The figure shows three views and two pictorial views of one solid part (mm, origin at its lowest corner). Answer the questions. A direction names the side the tool comes from. Round coordinates to 2 decimals unless told otherwise and drop trailing zeros. Write each loop counter-clockwise with the first axis right and the second up, starting at its lowest first coordinate (ties: lowest second). Pieces come first, ordered by that corner, then holes. Notation, with made-up numbers: (-2, -20) -> (14, -20) arc R27 cw to (14, 7) -> close; hole circle Ø2 at (60.25, -34.5). An arc over 180 degrees is marked (long way). One line per item, written item: value.
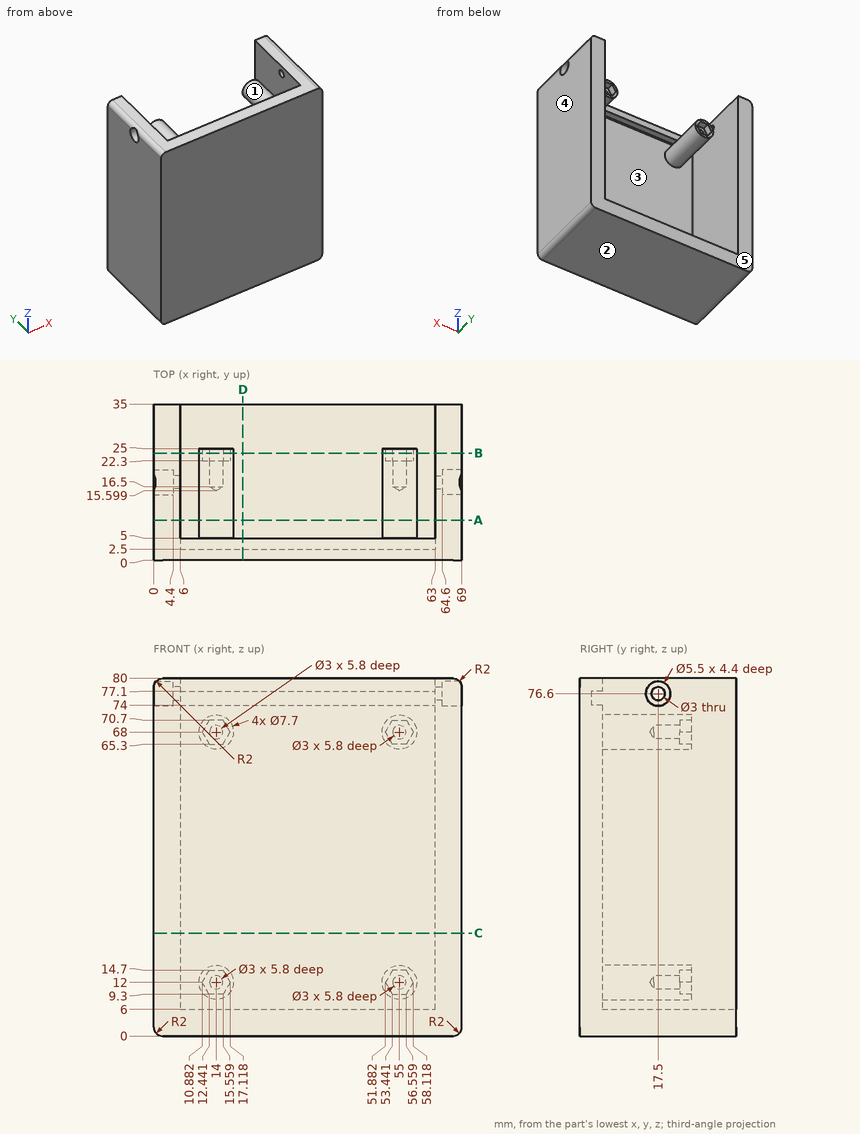
(1) Flat-ended cylindrical pins translate along their axes: pin 1 Ø5 at (y, z) = (17.5, 76.6) entering from -X; pin 2 Ø1.3 at (x, y) = (14.5, 23.5) entering from +Z; pin 3 Ø2.5 at (x, z) = (56.5, 66.5) entering from +Y. Find the tip coordinate at first contact, or state that the pin passes through.
Reported:
pin 1: stops at x = 4.4
pin 2: stops at z = 71.85
pin 3: stops at y = 25
(2) For a pull along X with two mould halves and no side action, classify the marked faces 3, 4 and 5 as pulls with the +X half, pulls with the -X half, needs draft (parallel to the pull), parting line crosses it, or undercut.
Reported:
face 3: undercut
face 4: pulls with the +X half
face 5: needs draft
(3) Find section B-B on y = 24. Give the number of separate pieces and of enclosed holes in the cut face, plus the area to 3 significant figures.
Reported:
separate pieces: 5
enclosed holes: 4
area: 1,380 mm2
(4) A tool of negligible diameter and unlimited length cuts with its end or side. For the marked faces 1 and 2, from which of +Z, -Z, +X, -X, +Y, -Y can it reach the whole face along a straight path? Write none if from no direction.
Reported:
face 1: +Y
face 2: -Z, +X, -X, +Y, -Y
(5) Find section A-A on y = 9. Give the vertices of the cut face in (x, z).
Reported:
outline: (0, 2) arc R2 ccw to (2, 0) -> (67, 0) arc R2 ccw to (69, 2) -> (69, 78) arc R2 ccw to (67, 80) -> (63, 80) -> (63, 6) -> (6, 6) -> (6, 80) -> (2, 80) arc R2 ccw to (0, 78) -> close; circle Ø7.7 at (14, 12); circle Ø7.7 at (14, 68); circle Ø7.7 at (55, 12); circle Ø7.7 at (55, 68)
(6) Find section C-C on z = 23. Give the vertices of the cut face in (x, y), plus the area to 3 significant figures.
Reported:
outline: (0, 0) -> (69, 0) -> (69, 35) -> (63, 35) -> (63, 5) -> (6, 5) -> (6, 35) -> (0, 35) -> close
area: 705 mm2
(7) Find section D-D on x = 20. Give the vertices of the cut face in (y, z), plus the area to 3 significant figures.
Reported:
outline: (0, 0) -> (35, 0) -> (35, 6) -> (5, 6) -> (5, 74) -> (2.5, 74) -> (2.5, 77.1) -> (5, 77.1) -> (5, 80) -> (0, 80) -> close
area: 572 mm2
(8) Consider probe 1 along X at (y, z) = (19.75, 68); probe 2 along X at (y, z) = (14, 50.5); probe 3 along Y at (x, z) = (1.85, 76.6). Determine where each line is inside the solid, lowest interval first.
Reported:
probe 1: x = 0 to 6, 10.15 to 12.5, 15.5 to 17.85, 51.15 to 53.5, 56.5 to 58.85, 63 to 69
probe 2: x = 0 to 6, 63 to 69
probe 3: y = 0 to 14.75, 20.25 to 35
